Work out the finished part from the listing and answer in its coordinate system (mm). Round coordinates to 2 decimals unless told otherwise and drop trailing zeros. Loops run counter-clockwise (first coordinate to the right, second up) from the corner with the lowest first, then second, coordinate; pieces in that order, holes last.
Autodesk Inventor part; units mm, degrees
ref_plane "YZ Plane" through (0, 0, 0) normal (1, 0, 0) x (0, 1, 0)
ref_plane "XZ Plane" through (0, 0, 0) normal (0, 1, 0) x (-1, 0, 0)
ref_plane "XY Plane" through (0, 0, 0) normal (0, 0, 1) x (1, 0, 0)
sketch "Sketch1" plane through (0, 0, 0) normal (0, 1, 0) x (-1, 0, 0)
  line L0 (70, -42.5) -> (-70, -42.5)
  line L1 (-70, -42.5) -> (-70, 42.5)
  line L2 (-70, 42.5) -> (70, 42.5)
  line L3 (70, 42.5) -> (70, -42.5)
  line L4 (70, -42.5) -> (-70, 42.5) construction
  line L5 (-70, -42.5) -> (70, 42.5) construction
  point P0 (0, 0)
  point P1 (0, 0)
  point P2 (0, 0)
  dimension "d0" = 140
  dimension "d1" = 85
extrude "Lid" add sketch "Sketch1" against normal blind 3
sketch "Sketch2" plane through (0, 0, 0) normal (0, 1, 0) x (-1, 0, 0)
  line L0 (29, 12) -> (-29, 12) construction
  line L1 (-29, 12) -> (-29, 35) construction
  line L2 (-29, 35) -> (29, 35) construction
  line L3 (29, 35) -> (29, 12) construction
  line L4 (29, 12) -> (-29, 35) construction
  line L5 (-29, 12) -> (29, 35) construction
  circle A0 centre (29, 12) radius 1.4
  circle A1 centre (-29, 12) radius 1.4
  circle A2 centre (-29, 35) radius 1.4
  circle A3 centre (29, 35) radius 1.4
  point P0 (0, 0)
  point P1 (0, 0)
  point P2 (0, 23.5)
  point P3 (0, 23.5)
  point P4 (0, 23.5)
  dimension "d4" = 23
  dimension "d5" = 58
  dimension "d6" = 12
  dimension "d7" = 2.8
extrude "M3_Mount_Holes" cut sketch "Sketch2" along normal through all both and the other way through all
equation "\"d1\" = 0.607143 * d0"
equation "\"d2\" = 0.0214286 * d0"
equation "\"d4\" = 0.164286 * d0"
equation "\"d5\" = 0.414286 * d0"
equation "\"d7\" = 0.02 * d0"
properties part number "Top-Lid" material "Polycarbonate, Clear"
Item 1: Section B-B, the plane z = 35 is taken. Give the vertices of the cut face in (x, y), plus the area to 3 significant figures.
Item 2: Section A-A, the plane x = 29 is taken. Give the vertices of the cut face in (y, z), plus the area to 3 significant figures.
Item 3: Determine the mould class of faces 1 (the face through (-28.82, -1.48, 36.39)), 2 (the face through (1, -3, 1)), 3 (the face through (-70, -1, 1)), 4 (the face through (70, -1, -1)) for opening direction X: pulls with the +X half, pulls with the -X half, needs draft (parallel to the pull), parting line crosses it, or undercut.
Item 4: Straight lines are drawn through the part: line 1 (Z direction, x = 29, y = -2.25); line 2 (Z direction, x = 29.5, y = -1.2). For each, find the intervals that lie inside material, in ascending order.
Item 5: This flat-tipped pin is pushed along its axis until it touches: P1, Ø2, axis at x = -29, z = 35, coming from the -Y side. Where does it stop, or does it pass through?
Answer below:
1. outline: (-70, -3) - (-30.4, -3) - (-30.4, 0) - (-70, 0) - close; (-27.6, -3) - (27.6, -3) - (27.6, 0) - (-27.6, 0) - close; (30.4, -3) - (70, -3) - (70, 0) - (30.4, 0) - close
1. area: 403 mm2
2. outline: (-3, -42.5) - (0, -42.5) - (0, 10.6) - (-3, 10.6) - close; (-3, 13.4) - (0, 13.4) - (0, 33.6) - (-3, 33.6) - close; (-3, 36.4) - (0, 36.4) - (0, 42.5) - (-3, 42.5) - close
2. area: 238 mm2
3. face 1: undercut
3. face 2: needs draft
3. face 3: pulls with the -X half
3. face 4: pulls with the +X half
4. line 1: z = -42.5 to 10.6, 13.4 to 33.6, 36.4 to 42.5
4. line 2: z = -42.5 to 10.69, 13.31 to 33.69, 36.31 to 42.5
5. P1: passes through
